Source: CAD feature listing. Evaluate the final solid. Frame: model axes, mm. A direction names the side the tool comes from. Give positions to 0.01 mm unless a question says otherwise; leave off trailing zeros. Order: outer loops, then holes, each group sorted by start corner. A loop starts at its lowest first (then second) coordinate and runs counter-clockwise, first axis right, second up. Notation, with made-up numbers: M -24,49.5 L -7,49.5 A24 cw -7,82.5 Z; hole C 39,17 d2. An arc over 180 degrees is marked long. Return JSON: item names as keys, results as strings.
from build123d import *

# Parameters (mm, degrees)
ESQUISSE1_W                  = 78
ESQUISSE1_H                  = 165
BOSS_EXTRU_2_DEPTH           = 250
ENL_V_MAT_EXTRU_6_DEPTH      = 359.895122211
ENL_V_MAT_EXTRU_6_DEPTH_BACK = 32
ENL_V_MAT_EXTRU_7_DEPTH      = 332.582217321
ENL_V_MAT_EXTRU_7_DEPTH_BACK = 78


with BuildPart() as part:
    # Esquisse1 → Boss.-Extru.2 (new body)
    with BuildSketch(Plane.XY):
        with Locations((-118.933346394, -120.878383423)):
            Rectangle(ESQUISSE1_W, ESQUISSE1_H)
    extrude(amount=BOSS_EXTRU_2_DEPTH)

    # Esquisse3 → Enlèv. mat.-Extru.6 (cut, two sides: drawn at the far end of the back side and taken through both)
    with BuildSketch(Plane.XY.offset(250).offset(-ENL_V_MAT_EXTRU_6_DEPTH_BACK)):
        Polygon((-83.933346394, -575.046739794), (-83.933346394, -203.378383423), (-83.933346394, -43.878383423), (-153.933346394, -43.878383423), (-153.933346394, -203.378383423), (-153.933346394, -575.046739794), (-153.933346394, -1318.383452535), (-83.933346394, -1318.383452535), align=None)
    extrude(amount=ENL_V_MAT_EXTRU_6_DEPTH + ENL_V_MAT_EXTRU_6_DEPTH_BACK, mode=Mode.SUBTRACT)

    # Esquisse5 → Enlèv. mat.-Extru.7 (cut, two sides: drawn at the far end of the back side and taken through both)
    with BuildSketch(Plane(origin=(-79.933346394, 0, 0), x_dir=(0, 0, -1), z_dir=(1, 0, 0)).offset(-ENL_V_MAT_EXTRU_7_DEPTH_BACK)):
        Polygon((-779.795226733, 193.681557603), (-250, -78.878383423), (-8, -203.378383423), (521.795226733, -475.938324449), (-23.324655319, -1535.528777915), (-1324.915108785, -865.908895863), align=None)
    extrude(amount=ENL_V_MAT_EXTRU_7_DEPTH + ENL_V_MAT_EXTRU_7_DEPTH_BACK, mode=Mode.SUBTRACT)


solid = part.part
1. Set-up query: faces 4 (the face through (-118, -43.878, 234)), 5 (the face through (-157.933, -104, 95)). Return all of +Z, -Z, +X, -X, +Y, -Y with unobstructed straight access to the full face (end or side cutting, diameter ignored); none if empty.
Evaluation:
{"face 4": "+Z, -Y", "face 5": "+Z, -Z, -X, +Y, -Y"}
2. First-contact query: pin 1 (2 mm diameter, centred on x = -124, y = -88.5, fed in from +Z); pin 2 (9.5 mm diameter, centred on x = -107, z = 240.5, fed in from -Y); pin 3 (4 mm diameter, centred on x = -104.5, z = 136.5, fed in from -Y). Flat tips, straight axial feed; report the tip coordinate or a pass-through.
Evaluation:
{"pin 1": "stops at z = 218", "pin 2": "stops at y = -43.88", "pin 3": "stops at y = -138.3"}
3. Section query B-B (y = -65.5). Return loops of the section in (x, z).
Evaluation:
{"outline": "M -157.93,0 L -79.93,0 L -79.93,250 L -83.93,250 L -83.93,218 L -153.93,218 L -153.93,250 L -157.93,250 Z"}
4. Ray query, probe 1 along Z at (x, y) = (-84, -87); probe 2 along Z at (x, y) = (-139.5, -181); probe 3 along Y at (x, z) = (-97, 162). Return the intervals inside material, ascending.
Evaluation:
{"probe 1": "z = 0 to 218", "probe 2": "z = 0 to 51.5", "probe 3": "y = -124.15 to -38.38"}
5. Draft query along X for faces 1 (the face through (-119.48, -142, 127.31)), 2 (the face through (-119, -69, 218)), 3 (the face through (-79.933, -104, 95)). Return one class per face: pulls with the +X half, pulls with the -X half, needs draft (parallel to the pull), parting line crosses it, or undercut.
Evaluation:
{"face 1": "needs draft", "face 2": "undercut", "face 3": "pulls with the +X half"}
6. Section query D-D (y = -136). Return loops of the section in (x, z).
Evaluation:
{"outline": "M -157.93,0 L -79.93,0 L -79.93,138.97 L -157.93,138.97 Z"}
7. Section query C-C (z = 28). Return loops of the section in (x, y), then the cut area to 3 significant figures.
Evaluation:
{"outline": "M -157.93,-193.09 L -79.93,-193.09 L -79.93,-38.38 L -157.93,-38.38 Z", "area": "12,100 mm^2"}
8. Section query A-A (x = -109). Return loops of the section in (y, z).
Evaluation:
{"outline": "M -203.38,0 L -38.38,0 L -38.38,250 L -43.88,250 L -43.88,218 L -95.34,218 L -203.38,8 Z"}
